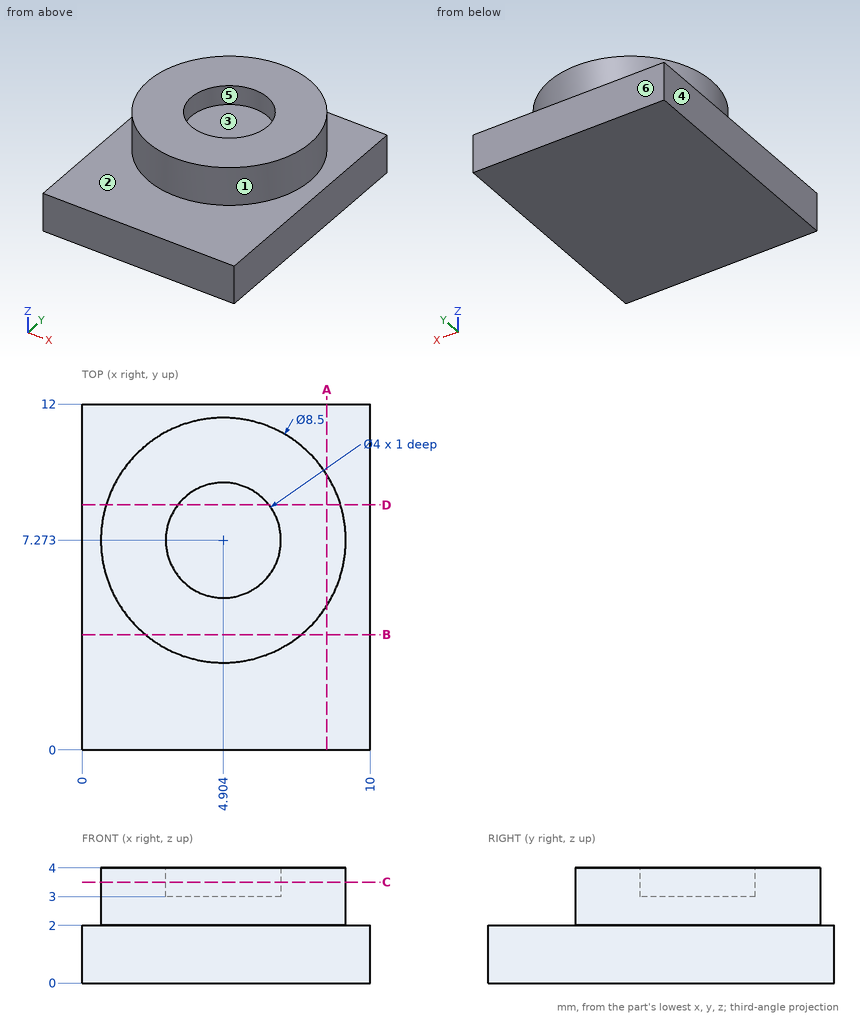
The figure shows three views and two pictorial views of one solid part (mm, origin at its lowest corner). Answer the questions. A direction names the side the tool comes from. Coordinates: 2 decimals unless noted, no trailing zeros. Write each loop counter-clockwise with the first axis right and the second up, starting at its lowest first coordinate (ties: lowest second). Pieces come first, ordered by that corner, then holes.
1. The part is cut by section D-D, the plane y = 8.5. Write down the section's boundary in (x, z) (1 decimal).
Results list:
outline: (0, 0) - (10, 0) - (10, 2) - (9, 2) - (9, 4) - (6.5, 4) - (6.5, 3) - (3.3, 3) - (3.3, 4) - (0.8, 4) - (0.8, 2) - (0, 2) - close
2. A flat-ended cylindrical pin translates along its axis: pin 1 (1 mm diameter, centred on x = 8, z = 3, fed in from +Y). Find the tip coordinate at first contact, or state that the pin passes through.
Results list:
pin 1: stops at y = 10.64
3. For a pull along X with two mould halves and no side action, classify the marked faces 1, 2, 3 and 4 as +X half, -X half, draft (parallel to the pull), parting line (faces both ways), or undercut.
Results list:
face 1: parting line
face 2: draft
face 3: undercut
face 4: -X half
4. Consider line 1 along Z through (x, y) = (7.5, 0.5); line 2 along Y through (x, z) = (5, 2.6); line 3 along X through (y, z) = (10.5, 3.2). Determine where each line is inside the solid, lowest interval first.
Results list:
line 1: z = 0 to 2
line 2: y = 3.02 to 11.52
line 3: x = 2.14 to 7.67
5. The part is cut by section C-C, the plane z = 3.5. Write down the section's boundary in (x, y), and give its area (3 significant figures).
Results list:
outline: circle Ø8.5 at (4.9, 7.27); hole circle Ø4 at (4.9, 7.27)
area: 44.2 mm2
6. The part is cut by section B-B, the plane y = 4. Write down the section's boundary in (x, z).
Results list:
outline: (0, 0) - (10, 0) - (10, 2) - (7.62, 2) - (7.62, 4) - (2.19, 4) - (2.19, 2) - (0, 2) - close
7. For the marked faces 5 and 6, determine the directions among +Z, -Z, +X, -X, +Y, -Y from which every point of the face is accessible in a straight line to the end or side of a thin tool.
Results list:
face 5: +Z
face 6: +Z, -Z, +X, -X, +Y
8. The part is cut by section A-A, the plane x = 8.5. Write down the section's boundary in (y, z).
Results list:
outline: (0, 0) - (12, 0) - (12, 2) - (9.54, 2) - (9.54, 4) - (5.01, 4) - (5.01, 2) - (0, 2) - close
